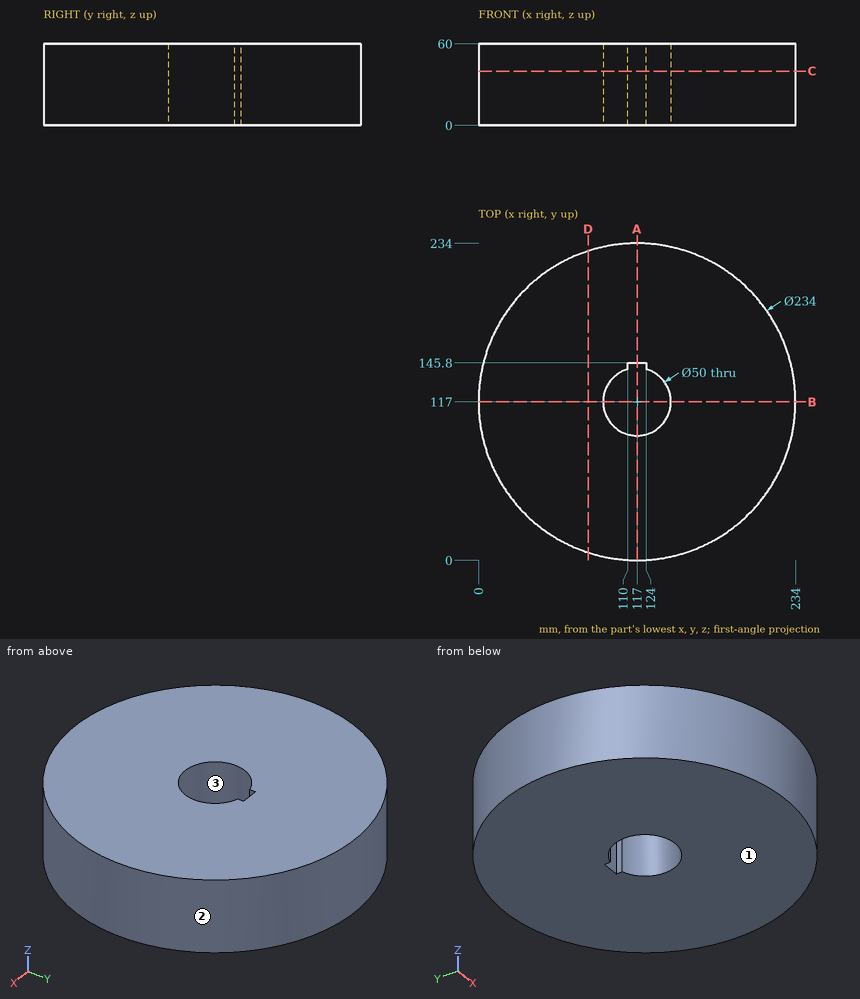
Geometry check sheet. Reference: drawing and pictorial views, mm from the part's lowest x, y, z. Give positions to 0.01 mm unless a question says otherwise; leave off trailing zeros. Loops run counter-clockwise (first coordinate to the right, second up) from the corner with the lowest first, then second, coordinate; pieces in that order, holes last. Notation, with made-up numbers: M 26,54 L 73,54 A27 cw 73,77 Z; hole C -26.5,21 d4. An arc over 180 degrees is marked long. Use a Markdown table: item, result. Add a question column.
Q1. Sectioned sample at C-C, the plane z = 40. Record the cut outline in (x, y), then the cut area to 3 significant figures.
Q2. Sectioned sample at A-A, the plane x = 117. Record the cut outline in (y, z).
Q3. Sectioned sample at D-D, the plane x = 81. Record the cut outline in (y, z), then the cut area to 3 significant figures.
Q4. Sectioned sample at B-B, the plane y = 117. Record the cut outline in (x, z).
Q5. Go/stop test with flat-tipped pins: pin 1 (3 mm diameter, centred on x = 184.5, z = 36, fed in from +Y); pin 2 (3 mm diameter, centred on y = 201, z = 47.5, fed in from -X); pin 3 (2 mm diameter, centred on x = 94.5, z = 21, fed in from +Y). Record where each tip stops, or that it passes through.
Q6. Scan lines: line 1 along Y through (x, z) = (117, 27); line 2 along X through (y, z) = (113, 6.5); line 3 along Y through (x, z) = (87, 16). Record each from-to range of solid material in increasing order. Write a range as [from, to].
Q7. Mould release check, pull along Y, two halves, no side actions. Record for the marked faces 1, 2 and 3: pulls with the +Y half, pulls with the -Y half, needs draft (parallel to the pull), parting line crosses it, or undercut.
Verdict:
| question | item | result |
|---|---|---|
| 1 | outline | C 117,117 d234; hole M 110,141 A25 ccw long 124,141 L 124,145.8 L 110,145.8 Z |
| 1 | area | 41,000 mm^2 |
| 2 | outline | M 0,0 L 92,0 L 92,60 L 0,60 Z; M 145.8,0 L 234,0 L 234,60 L 145.8,60 Z |
| 3 | outline | M 5.68,0 L 228.32,0 L 228.32,60 L 5.68,60 Z |
| 3 | area | 13,400 mm^2 |
| 4 | outline | M 0,0 L 92,0 L 92,60 L 0,60 Z; M 142,0 L 234,0 L 234,60 L 142,60 Z |
| 5 | pin 1 | y = 213.61 |
| 5 | pin 2 | x = 34.04 |
| 5 | pin 3 | y = 232.01 |
| 6 | line 1 | [0, 92], [145.8, 234] |
| 6 | line 2 | [0.07, 92.32], [141.68, 233.93] |
| 6 | line 3 | [3.91, 230.09] |
| 7 | face 1 | needs draft |
| 7 | face 2 | parting line crosses it |
| 7 | face 3 | undercut |
